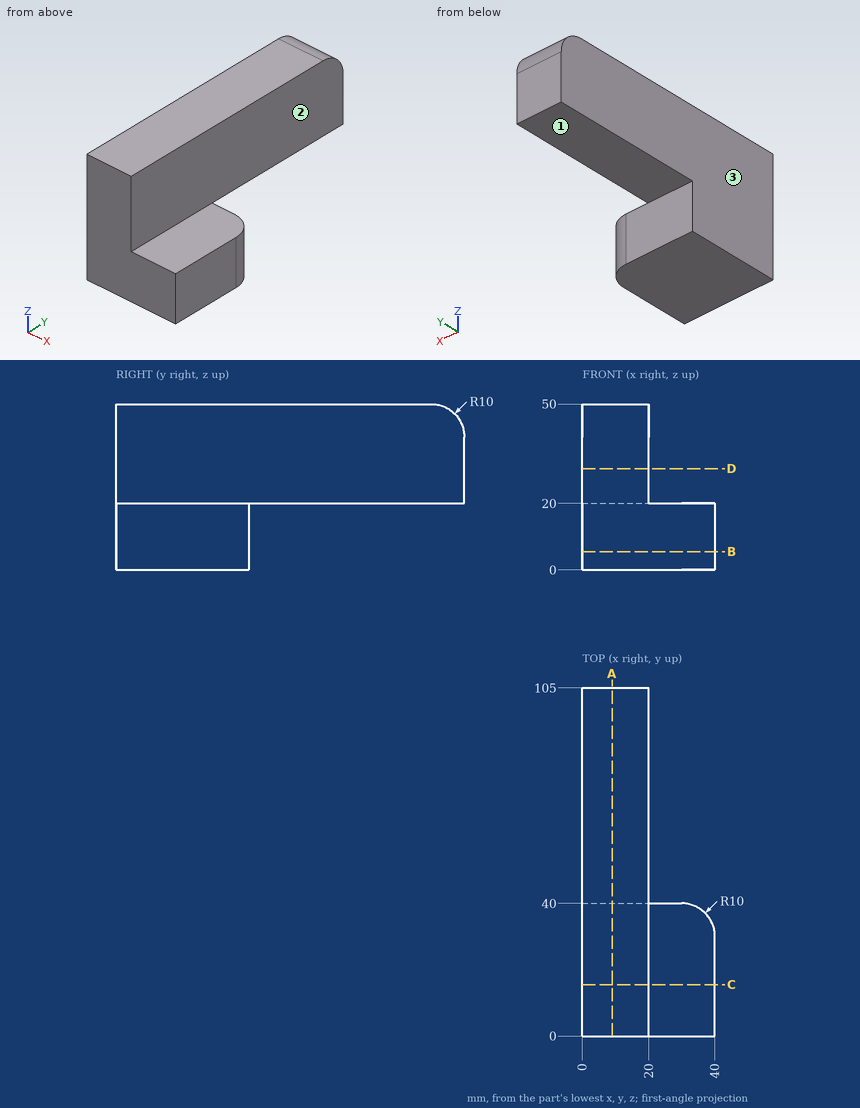
Here's the drawing with two shaded views (mm, measured from the low corner). I have some questions. A direction names the side the tool comes from. Round coordinates to 2 decimals unless told otherwise and drop trailing zeros. Order: outer loops, then holes, each group sorted by start corner. A loop starts at its lowest first (then second) coordinate and runs counter-clockwise, first axis right, second up. Notation, with made-up numbers: (35.25, -34.5) -> (48.25, -34.5) arc R16 cw to (48.25, -13.5) -> close; hole circle Ø7 at (30.5, 52). An arc over 180 degrees is marked (long way). Use a Markdown table: item, result. Add a question column.
(1) I need wall thicknesses on line 1 along X through (y, z) = (16.5, 37); line 2 along Z through (x, y) = (8, 53.5); line 3 along Y through (x, z) = (11, 40.5). Which ranges of each line are inside material? Lowest first, please.
(2) Suppose I cut it at C-C, the plane y = 15.5. Please give me the cut outline in (x, z), and give its area (3 significant figures).
(3) Suppose I cut it at B-B, the plane z = 5.5. Please give me the cut outline in (x, y), and give its area (3 significant figures).
(4) Suppose I cut it at D-D, the plane z = 30.5. Please give me the cut outline in (x, y), and give its area (3 significant figures).
(5) Suppose I cut it at A-A, the plane x = 9. Please give me the cut outline in (y, z), and give its area (3 significant figures).
(6) For the marked faces 1, 2 and 3, which set-ups out of +Z, -Z, +X, -X, +Y, -Y let a thin tool reach every point of the face, with its end or its side?
(7) For pin 1 Ø10 at (x, z) = (9.5, 7.5) entering from +Y; pin 2 Ø5 at (y, z) = (61.5, 32) entering from +X; pin 3 Ø22 at (x, y) = (8, 69) entering from -Z, each with a flat end and sliding along its axis, tell me the tip position at first contact or that it passes through.
Verdict:
| question | item | result |
|---|---|---|
| 1 | line 1 | 0 to 20 |
| 1 | line 2 | 20 to 50 |
| 1 | line 3 | 0 to 104.99 |
| 2 | outline | (0, 0) -> (40, 0) -> (40, 20) -> (20, 20) -> (20, 50) -> (0, 50) -> close |
| 2 | area | 1,400 mm2 |
| 3 | outline | (0, 0) -> (40, 0) -> (40, 30) arc R10 ccw to (30, 40) -> (0, 40) -> close |
| 3 | area | 1,580 mm2 |
| 4 | outline | (0, 0) -> (20, 0) -> (20, 105) -> (0, 105) -> close |
| 4 | area | 2,100 mm2 |
| 5 | outline | (0, 0) -> (40, 0) -> (40, 20) -> (105, 20) -> (105, 40) arc R10 ccw to (95, 50) -> (0, 50) -> close |
| 5 | area | 3,930 mm2 |
| 6 | face 1 | -Z, +X, -X, +Y |
| 6 | face 2 | +Z, +X, +Y, -Y |
| 6 | face 3 | +Z, -Z, -X, +Y, -Y |
| 7 | pin 1 | y = 40 |
| 7 | pin 2 | x = 20 |
| 7 | pin 3 | z = 20 |
